from build123d import *

# Parameters (mm, degrees)
F1_DEPTH    = 17.4625
F2_T2_ANGLE = 17.1649477786


# Not quite as in the source:
# - a fillet or chamfer that OpenCascade refuses, or shapes differently, is made with other operations: its cross-section is extruded or revolved along the edge and cut away or added


with BuildPart() as f1:
    # F0 (on Front) → F1 (new body)
    with BuildSketch(Plane.XZ):
        with BuildLine():
            Line((0, 87.3125), (0, 0))
            Line((0, 0), (25.4, 0))
            ThreePointArc((25.4, 0), (152.4, 6.35), (279.4, 0))
            Line((279.4, 0), (304.8, 0))
            Line((304.8, 0), (304.8, 87.3125))
            Line((304.8, 87.3125), (0, 87.3125))
        make_face()
    extrude(amount=F1_DEPTH)

    # F2: fillet of radius 5.08 on 1 edges, made by hand

    # F2_s1 → F2_t2 (revolve, cut)
    with BuildSketch(Plane(origin=(-37.9289804695, 0, -5.7243521326), x_dir=(0, 1, 0), z_dir=(-0.9888020759, 0, -0.1492328874))):
        with BuildLine():
            ThreePointArc((-12.3825, 2.2072818505), (-15.9746024484, 0.7193842989), (-17.4625, -2.8727181495))
            Line((-17.4625, -2.8727181495), (-17.4625, 2.2072818505))
            Line((-17.4625, 2.2072818505), (-12.3825, 2.2072818505))
        make_face()
    revolve(axis=Axis((152.4, -17.4625, -1266.8250000001), (0, 1, 0)), revolution_arc=F2_T2_ANGLE, mode=Mode.SUBTRACT)


solid = f1.part
Geometry check sheet. Reference: the model listing, model coordinates, mm. Round coordinates to 2 decimals unless told otherwise and drop trailing zeros.
Item 1: Go/stop test with a flat-tipped pin: pin 1 Ø12 at (x, z) = (155.5, 75) entering from +Y. Record where the tip stops, or that it passes through.
Determined:
pin 1: stops at y = 0
Item 2: Mould release check, pull along X, two halves, no side actions. Record for faces 1 (the face through (150.62, -6.1, 6.35)), 2 (the face through (0, -9, 44)), 3 (the face through (304.8, -9, 43)), 4 (the face through (150, 0, 44)): +X half, -X half, draft (parallel to the pull), parting line (faces both ways), or undercut.
Determined:
face 1: undercut
face 2: -X half
face 3: +X half
face 4: draft
Item 3: Material ranges on line 1 along Z through (x, y) = (232.5, -2.5); line 2 along Z through (x, y) = (152.5, -16), recorded low to high.
Determined:
line 1: z = 3.83 to 87.31
line 2: z = 7.86 to 87.31
